The listing builds one solid part. Answer for the finished solid, in the listing's coordinates (mm). Face numbers are marked on the shaded views. A direction names the side the tool comes from. Give positions to 0.01 mm unless a question says otherwise; leave off trailing zeros. Order: outer loops, then holes, each group sorted by start corner. A loop starts at its lowest first (then second) coordinate and runs counter-clockwise, first axis right, second up. Notation, with made-up numbers: (19, 49) - (45, 49) arc R20 ccw to (45, 55) - close; hole circle Ø9 at (89.5, 13). An arc over 180 degrees is marked (long way). Answer as a JSON object with one key per item and string values. Group by question number.
Q1. A cutting plane is placed at D-D, the plane x = 6.25. Give the vertices of the cut face in (y, z).
Q2. The mould has two halves that part along Y. Classify the marked faces 4 and 5: released by +Y, released by -Y, zero draft, split by the parting line, or undercut.
Q3. A cutting plane is placed at B-B, the plane x = 7.5. Give the vertices of the cut face in (y, z), and give its area (3 significant figures).
Q4. A cutting plane is placed at C-C, the plane y = -1.25. Give the vertices of the cut face in (x, z), and give its area (3 significant figures).
Q5. Consider line 1 (Y direction, x = 3.2, z = 0); line 2 (Y direction, x = 4, z = -2.75). Determine where each line is inside the solid, lowest interval first.
Q6. A cutting plane is placed at A-A, the plane z = 0. Give the vertices of the cut face in (x, y), and give its area (3 significant figures).
Q7. For the marked faces 1, 2 and 3, determine the directions among +Z, -Z, +X, -X, +Y, -Y from which every point of the face is accessible in a straight line to the end or side of a thin tool.
Q8. Given pin 1 (1.5 mm diameter, centred on x = 3, y = -2.5, fed in from +Z); pin 2 (1.2 mm diameter, centred on x = 7.5, y = -0.5, fed in from +Z); pin 3 (0.5 mm diameter, centred on y = 3, z = -1, fed in from +X), each flat-ended and moving along its own axis, determine where each tip first touches the part or whether it passes through.
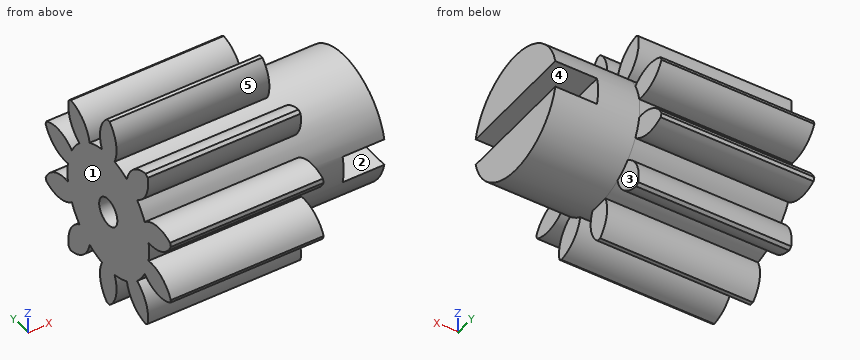
from build123d import *
from build123d.topology import SkipClean

# Parameters (mm, degrees)
BASPROSKE_W         = 5.5
BASPROSKE_H         = 3.6
TOOTHCUT_DEPTH      = 8.494664769
TEETHCUTS_COUNT     = 10
TEETHCUTS_ANGLE     = 324
BORSKE_R            = 0.5
BORE_DEPTH          = 50.0000508
SKETCH_1_R          = 2.249
SKETCH_1_R_2        = 0.5
EXTRUDE_1_DEPTH     = 3
CUT_EXTRUDE_START   = -1.5
CUT_EXTRUDE_1_DEPTH = 1.5


with BuildPart() as part:
    # BasProSke → Base-Revolve (revolve)
    with BuildSketch(Plane(origin=(0, 0, 0), x_dir=(1, 0, 0), z_dir=(0, 1, 0)), mode=Mode.PRIVATE) as base_revolve_sk:
        with Locations((2.75, 1.8)):
            Rectangle(BASPROSKE_W, BASPROSKE_H)
    revolve(base_revolve_sk.sketch.rotate(Axis((-10, 0, 0), (1, 0, 0)), 180), axis=Axis((-10, 0, 0), (1, 0, 0)))

    # TooCutSke → ToothCut (cut, through all)
    with BuildSketch(Plane(origin=(0, 0, 0), x_dir=(0, 0, -1), z_dir=(1, 0, 0))):
        with BuildLine():
            ThreePointArc((0.355978269, 2.22064866), (0, 2.249), (-0.355978269, 2.22064866))
            ThreePointArc((-0.355978269, 2.22064866), (-0.512117582, 2.960985626), (-1.080212515, 3.460732015))
            ThreePointArc((-1.080212515, 3.460732015), (0, 3.6254), (1.080212515, 3.460732015))
            ThreePointArc((1.080212515, 3.460732015), (0.512117582, 2.960985626), (0.355978269, 2.22064866))
        make_face()
    toothcut = extrude(amount=TOOTHCUT_DEPTH, mode=Mode.SUBTRACT)

    # TeethCuts: ToothCut ×10 about axis
    teethcuts_axis = Axis((-10, 0, 0), (1, 0, 0))
    for i in range(1, TEETHCUTS_COUNT):
        add(toothcut.rotate(teethcuts_axis, i * TEETHCUTS_ANGLE / (TEETHCUTS_COUNT - 1)), mode=Mode.SUBTRACT)

    # BorSke → Bore (cut, symmetric)
    with BuildSketch(Plane(origin=(0, 0, 0), x_dir=(0, 0, -1), z_dir=(1, 0, 0))):
        with Locations(Location((0, 0, 0), (0, 0, 180))):
            Circle(BORSKE_R)
    extrude(amount=BORE_DEPTH, both=True, mode=Mode.SUBTRACT)

    # Sketch 1 → Extrude 1 (add)
    with SkipClean():  # the faces are left unmerged after this step: merging them gives an invalid solid
        with BuildSketch(Plane(origin=(5.5, 0, 0), x_dir=(0, 0, -1), z_dir=(1, 0, 0))):
            with Locations(Location((0, 0, 0), (0, 0, 171.107244316))):
                Circle(SKETCH_1_R)
            Circle(SKETCH_1_R_2, mode=Mode.SUBTRACT)
        extrude(amount=EXTRUDE_1_DEPTH)
    add(part.part.scale(1), mode=Mode.REPLACE)  # the faces are merged on a copy

    # Sketch 2 → Cut-Extrude 1 (cut)
    with BuildSketch(Plane(origin=(8.5, 0, 0), x_dir=(0, 0, -1), z_dir=(1, 0, 0)).offset(CUT_EXTRUDE_START)):
        with BuildLine():
            Line((-0.5, 0), (-0.5, -2.19271544))
            ThreePointArc((-0.5, -2.19271544), (0, -2.249), (0.5, -2.19271544))
            Line((0.5, -2.19271544), (0.5, 0))
            Line((0.5, 0), (0.5, 2.19271544))
            ThreePointArc((0.5, 2.19271544), (0, 2.249), (-0.5, 2.19271544))
            Line((-0.5, 2.19271544), (-0.5, 0))
        make_face()
    extrude(amount=CUT_EXTRUDE_1_DEPTH, mode=Mode.SUBTRACT)


solid = part.part
Reply:
{
 "1": {"outline": "circle Ø4.5 at (0, 0); hole circle Ø1 at (0, 0)"},
 "2": {"face 4": "zero draft", "face 5": "undercut"},
 "3": {"outline": "(-2.19, -0.5) arc R2.25 ccw to (2.19, -0.5) - close; (-2.19, 0.5) - (2.19, 0.5) arc R2.25 ccw to start", "area": "11.4 mm^2"},
 "4": {"outline": "(0, -2.49) - (5.5, -2.49) - (5.5, -1.87) - (8.5, -1.87) - (8.5, -0.5) - (7, -0.5) - (7, 0.5) - (8.5, 0.5) - (8.5, 1.87) - (5.5, 1.87) - (5.5, 2.49) - (0, 2.49) - close", "area": "37.2 mm^2"},
 "5": {"line 1": "y = -2.25 to -0.5, 0.5 to 2.25", "line 2": "y = -2.19 to -1.52, -0.46 to 0.46, 1.52 to 2.19"},
 "6": {"outline": "(0, -2.25) - (7, -2.25) - (7, -0.5) - (0, -0.5) - close; (0, 0.5) - (7, 0.5) - (7, 2.25) - (0, 2.25) - close", "area": "24.5 mm^2"},
 "7": {"face 1": "+Z, -Z, -X, +Y, -Y", "face 2": "+X, +Y, -Y", "face 3": "-Z, +X, +Y"},
 "8": {"pin 1": "stops at z = 2.95", "pin 2": "stops at z = 2.25", "pin 3": "stops at x = 5.5"}
}
